Autodesk Inventor part; units mm, degrees
ref_plane "YZ Plane" through (0, 0, 0) normal (1, 0, 0) x (0, 1, 0)
ref_plane "XZ Plane" through (0, 0, 0) normal (0, 1, 0) x (-1, 0, 0)
ref_plane "XY Plane" through (0, 0, 0) normal (0, 0, 1) x (1, 0, 0)
sketch "Sketch1" plane through (0, 0, 0) normal (0, 1, 0) x (-1, 0, 0)
  line L0 (0, 0) -> (63.5, 0)
  line L1 (63.5, 0) -> (63.5, -38.1)
  line L2 (63.5, -38.1) -> (0, -38.1)
  line L3 (0, -38.1) -> (0, 0)
  dimension "d0" = 63.5
  dimension "d1" = 38.1
extrude "Extrusion1" add sketch "Sketch1" along normal blind 6.35
sketch "Sketch2" plane through (0, 6.35, 0) normal (0, 1, 0) x (1, 0, 0)
  line L0 (-63.5, 0) -> (0, 0)
  line L1 (0, 0) -> (0, 38.1)
  line L2 (0, 38.1) -> (-63.5, 38.1)
  line L3 (-63.5, 38.1) -> (-63.5, 0)
  line L4 (0, 0) -> (0, 38.1) construction
  line L5 (0, 19.05) -> (-31.75, 19.05) construction
  circle A0 centre (-31.75, 19.05) radius 3.175
  dimension "d4" = 31.75
  dimension "d5" = 90
  dimension "d6" = 6.35
extrude "Extrusion2" cut sketch "Sketch2" against normal blind 6.35 contours A0
sketch "Sketch3" plane through (0, 0, 0) normal (0, -1, 0) x (1, 0, 0)
  circle A0 centre (-31.75, -19.05) radius 3.175
  line L0 (0, 0) -> (-63.5, 0)
  line L1 (-63.5, 0) -> (-63.5, -38.1)
  line L2 (-63.5, -38.1) -> (0, -38.1)
  line L3 (0, -38.1) -> (0, 0)
  line L4 (-31.75, -19.05) -> (-19.05, -19.05) construction
  line L5 (-19.05, -19.05) -> (-19.05, 12.7) construction
  line L6 (-19.05, 12.7) -> (-19.05, -50.8) construction
  line L7 (-19.05, 12.7) -> (-44.45, 12.7)
  line L8 (-44.45, 12.7) -> (-44.45, -3.175)
  line L9 (-44.45, -3.175) -> (-19.05, -3.175)
  line L10 (-19.05, -3.175) -> (-19.05, 12.7)
  circle A1 centre (-31.75, -19.05) radius 3.175 construction
  line L11 (-31.75, -19.05) -> (-31.75, 6.35) construction
  line L12 (-31.75, -19.05) -> (-6.35, -19.05) construction
  circle A2 centre (-31.75, 6.35) radius 1.5875
  line L13 (-19.05, -19.05) -> (-19.05, -50.8) construction
  line L14 (-19.05, -50.8) -> (-19.05, 12.7) construction
  line L15 (-19.05, -50.8) -> (-44.45, -50.8)
  line L16 (-44.45, -50.8) -> (-44.45, -34.925)
  line L17 (-44.45, -34.925) -> (-19.05, -34.925)
  line L18 (-19.05, -34.925) -> (-19.05, -50.8)
  circle A3 centre (-31.75, -44.45) radius 1.5875
  dimension "d9" = 12.7
  dimension "d10" = 31.75
  dimension "d11" = 63.5
  dimension "d12" = 25.4
  dimension "d13" = 15.875
  dimension "d14" = 25.4
  dimension "d15" = 90
  dimension "d16" = 3.175
extrude "Extrusion3" add sketch "Sketch3" along normal blind 6.35 and the other way blind 3.175 contours L10 L9 L8 L0 | L0 L8 L7 L10 | L18 L15 L16 L2 | L2 L16 L17 L18
properties part number "mount"
Check sheet for the modelled part. Datum: model origin and axes. Units: mm. A direction names the side the tool comes from. Give positions to 0.01 mm unless a question says otherwise; leave off trailing zeros. Loops run counter-clockwise (first coordinate to the right, second up) from the corner with the lowest first, then second, coordinate; pieces in that order, holes last. Notation, with made-up numbers: M 56,28 L 106,28 A32 cw 106,64 Z; hole C 41,-29.5 d9. An arc over 180 degrees is marked long. Answer as a JSON object with one key per item and string values. Group by question number.
Q1. Material ranges on line 1 along Z through (x, y) = (-31.75, 1) (1 decimal); line 2 along Z through (x, y) = (-31.75, -0.75) (1 decimal); line 3 along Z through (x, y) = (-24.5, -2.5) (3 decimals), recorded low to high. Write a range as [from, to].
Q2. Release check for a two-part mould opening along X. For faces 4 (the flat face through (-32, -6.35, 3)), 5 (the cylindrical face through (-30.3, -1.5, 7)), 6 (the flat face through (-63.5, 3, -19)) record: released by +X, released by -X, zero draft, split by the parting line, or undercut.
Q3. Cross-section at B-B on y = -0.75. Give the number of separate pieces and of enclosed holes in the cut face, then the cut area to 3 significant figures.
Q4. Cross-section at C-C on z = -19.05. Record the cut outline in (x, y) (3 decimals), then the cut area to 3 significant figures.
Q5. Cross-section at D-D on x = -37. Record the cut outline in (y, z) (3 decimals).
Q6. Go/stop test with flat-tipped pins: P1, Ø1, axis at x = -13.5, z = -24, coming from the -Y side; P2, Ø1.5, axis at x = -40, z = -39, coming from the +Y side (3 decimals); P3, Ø4, axis at y = -3, z = 0.5, coming from the +X side; P4, Ø5, axis at x = -22, y = 4.5, coming from the +Z side. Record where each tip stops, or that it passes through.
Q7. Access from +Z, -Z, +X, -X, +Y, -Y to the whole of each face (thin tool, end or side, straight path). Record for faces 1 (the flat face through (-32, -3, -34.925)), 2 (the flat face through (-32, 3.175, 4)), 3 (the flat face through (-35, 3.175, -44)).
Evaluation:
{
 "1": {"line 1": "z = [-50.8, -46], [-42.9, -22.2], [-15.9, 4.8], [7.9, 12.7]", "line 2": "z = [-50.8, -46], [-42.9, -34.9], [-3.2, 4.8], [7.9, 12.7]", "line 3": "z = [-50.8, -34.925], [-3.175, 12.7]"},
 "2": {"face 4": "zero draft", "face 5": "undercut", "face 6": "released by -X"},
 "3": {"separate pieces": "2", "enclosed holes": "2", "area": "791 mm2"},
 "4": {"outline": "M -63.5,0 L -34.925,0 L -34.925,6.35 L -63.5,6.35 Z; M -28.575,0 L 0,0 L 0,6.35 L -28.575,6.35 Z", "area": "363 mm2"},
 "5": {"outline": "M -6.35,-50.8 L 3.175,-50.8 L 3.175,-38.1 L 6.35,-38.1 L 6.35,0 L 3.175,0 L 3.175,12.7 L -6.35,12.7 L -6.35,-3.175 L 0,-3.175 L 0,-34.925 L -6.35,-34.925 Z"},
 "6": {"P1": "stops at y = 0", "P2": "stops at y = 3.175", "P3": "stops at x = -19.05", "P4": "stops at z = 12.7"},
 "7": {"face 1": "+X, -X, -Y", "face 2": "+Z, +X, -X, +Y", "face 3": "-Z, +X, -X, +Y"}
}
